from build123d import *
from build123d.topology import SkipClean

# Parameters (mm, degrees)
SKETCH1_R               = 21
BOSS_EXTRUDE1_DEPTH     = 1.5
SKETCH2_R               = 2.65
CUT_EXTRUDE1_DEPTH      = 1.5
SKETCH5_W               = 10
SKETCH5_H               = 30
BOSS_EXTRUDE2_DEPTH     = 1.5
CIRPATTERN1_DEPTH       = 1.5
CUT_EXTRUDE4_REACH      = 38.65
SKETCH4_R               = 1.65
CUT_EXTRUDE5_REACH      = 38.742
SKETCH6_R               = 1.5
CUT_EXTRUDE6_DEPTH      = 37.650375169
CUT_EXTRUDE6_DEPTH_BACK = 37.650375169


# Read off the part's stored shape, not the designer's step: CirPattern1
with BuildPart() as part:
    # Sketch1 → Boss-Extrude1 (new, symmetric)
    with BuildSketch(Plane(origin=(0, 0, 0), x_dir=(1, 0, 0), z_dir=(0, 1, 0))):
        with Locations(Location((0, 0, 0), (0, 0, 270))):
            Circle(SKETCH1_R)
    extrude(amount=BOSS_EXTRUDE1_DEPTH, both=True)

    # Sketch2 → Cut-Extrude1 (cut)
    with BuildSketch(Plane(origin=(0, 1.5, 0), x_dir=(1, 0, 0), z_dir=(0, 1, 0))):
        with Locations((0, -15)):
            Circle(SKETCH2_R)
        with BuildLine():
            ThreePointArc((-2.65, -15), (0, -12.35), (2.65, -15))
            Line((2.65, -15), (4.067821782, -0.821782178))
            ThreePointArc((4.067821782, -0.821782178), (0, -4.15), (-4.067821782, -0.821782178))
            Line((-4.067821782, -0.821782178), (-2.65, -15))
        make_face()
        with BuildLine():
            ThreePointArc((-4.067821782, -0.821782178), (0, -4.15), (4.067821782, -0.821782178))
            Line((4.067821782, -0.821782178), (4.15, 0))
            ThreePointArc((4.15, 0), (0, 4.15), (-4.15, 0))
            Line((-4.15, 0), (-4.067821782, -0.821782178))
        make_face()
    cut_extrude1 = extrude(amount=-CUT_EXTRUDE1_DEPTH, mode=Mode.SUBTRACT)

    # Sketch5 → Boss-Extrude2 (add, symmetric)
    with BuildSketch(Plane(origin=(0, 0, 0), x_dir=(1, 0, 0), z_dir=(0, 1, 0))):
        with Locations((0, -15)):
            Rectangle(SKETCH5_W, SKETCH5_H)
    extrude(amount=BOSS_EXTRUDE2_DEPTH, both=True)

    # Mirror1: Cut-Extrude1 across plane
    with SkipClean():  # the faces are left unmerged after this step: merging them gives an invalid solid
        add(cut_extrude1.mirror(Plane.XY), mode=Mode.SUBTRACT)

    # CirPattern1 outline → CirPattern1 (cut)
    with BuildSketch(Plane(origin=(0, 0, 0), x_dir=(1, 0, 0), z_dir=(0, 1, 0))):
        with BuildLine():
            Line((3.772727273, -3.772727273), (15, -2.65))
            ThreePointArc((15, -2.65), (17.65, 0), (15, 2.65))
            Line((15, 2.65), (3.772727273, 3.772727273))
            Line((3.772727273, 3.772727273), (4.067821782, 0.821782178))
            ThreePointArc((4.067821782, 0.821782178), (0, -4.15), (-4.067821782, 0.821782178))
            Line((-4.067821782, 0.821782178), (-3.772727273, 3.772727273))
            Line((-3.772727273, 3.772727273), (-15, 2.65))
            ThreePointArc((-15, 2.65), (-17.65, 0), (-15, -2.65))
            Line((-15, -2.65), (-3.772727273, -3.772727273))
            Line((-3.772727273, -3.772727273), (-2.65, -15))
            ThreePointArc((-2.65, -15), (0, -17.65), (2.65, -15))
            Line((2.65, -15), (3.772727273, -3.772727273))
        make_face()
    extrude(amount=CIRPATTERN1_DEPTH, mode=Mode.SUBTRACT)

    # Sketch4 → Cut-Extrude4 (cut, up to next)
    with BuildSketch(Plane(origin=(0, 0, 0), x_dir=(1, 0, 0), z_dir=(0, 1, 0)), mode=Mode.PRIVATE) as cut_extrude4_sk1:
        with Locations(Location((0, 0, 0), (0, 0, 270))):
            Circle(SKETCH4_R)
    cut_extrude4_tool1 = extrude(cut_extrude4_sk1.sketch, amount=-CUT_EXTRUDE4_REACH, mode=Mode.PRIVATE) & part.part
    add(cut_extrude4_tool1.solids().sort_by_distance((0, 0, 0))[0], mode=Mode.SUBTRACT)

    # Sketch6 → Cut-Extrude5 (cut, up to next)
    with BuildSketch(Plane(origin=(0, 1.5, 0), x_dir=(1, 0, 0), z_dir=(0, 1, 0)), mode=Mode.PRIVATE) as cut_extrude5_sk1:
        with Locations(Location((2.5, -25.5, 0), (0, 0, 270))):
            Circle(SKETCH6_R)
    cut_extrude5_tool1 = extrude(cut_extrude5_sk1.sketch, amount=-CUT_EXTRUDE5_REACH, mode=Mode.PRIVATE) & part.part
    # Sketch6 → Cut-Extrude5 (cut, up to next)
    with BuildSketch(Plane(origin=(0, 1.5, 0), x_dir=(1, 0, 0), z_dir=(0, 1, 0)), mode=Mode.PRIVATE) as cut_extrude5_sk2:
        with Locations(Location((-2.5, -25.5, 0), (0, 0, 270))):
            Circle(SKETCH6_R)
    cut_extrude5_tool2 = extrude(cut_extrude5_sk2.sketch, amount=-CUT_EXTRUDE5_REACH, mode=Mode.PRIVATE) & part.part
    add(cut_extrude5_tool1.solids().sort_by_distance((2.5, 1.5, 25.5))[0], mode=Mode.SUBTRACT)
    add(cut_extrude5_tool2.solids().sort_by_distance((-2.5, 1.5, 25.5))[0], mode=Mode.SUBTRACT)

    # Sketch7 → Cut-Extrude6 (cut, two sides: drawn at the far end of the back side and taken through both)
    with BuildSketch(Plane(origin=(0, 0, 0), x_dir=(1, 0, 0), z_dir=(0, 1, 0)).offset(-CUT_EXTRUDE6_DEPTH_BACK)):
        with BuildLine():
            ThreePointArc((5, -20.396078054), (0, 21), (-5, -20.396078054))
            Line((-5, -20.396078054), (-5.519486194, -16.207382355))
            ThreePointArc((-5.519486194, -16.207382355), (-5.607043009, -15.695391034), (-5.647210443, -15.177522436))
            Line((-5.647210443, -15.177522436), (-6.513602442, -6.513602442))
            Line((-6.513602442, -6.513602442), (-15.177522436, -5.647210443))
            ThreePointArc((-15.177522436, -5.647210443), (-20.65, 0), (-15.177522436, 5.647210443))
            Line((-15.177522436, 5.647210443), (-6.513602442, 6.513602442))
            Line((-6.513602442, 6.513602442), (-5.647210443, 15.177522436))
            ThreePointArc((-5.647210443, 15.177522436), (0, 20.65), (5.647210443, 15.177522436))
            Line((5.647210443, 15.177522436), (6.513602442, 6.513602442))
            Line((6.513602442, 6.513602442), (15.177522436, 5.647210443))
            ThreePointArc((15.177522436, 5.647210443), (20.65, 0), (15.177522436, -5.647210443))
            Line((15.177522436, -5.647210443), (6.513602442, -6.513602442))
            Line((6.513602442, -6.513602442), (5.647210443, -15.177522436))
            ThreePointArc((5.647210443, -15.177522436), (5.607043009, -15.695391034), (5.519486194, -16.207382355))
            Line((5.519486194, -16.207382355), (5, -20.396078054))
        make_face()
    extrude(amount=CUT_EXTRUDE6_DEPTH + CUT_EXTRUDE6_DEPTH_BACK, mode=Mode.SUBTRACT)


solid = part.part
Can you work these out from the model? Positions are in its coordinate system, mm. A direction names the side the tool comes from. Round coordinates to 2 decimals unless told otherwise and drop trailing zeros. Order: outer loops, then holes, each group sorted by start corner. A loop starts at its lowest first (then second) coordinate and runs counter-clockwise, first axis right, second up. Notation, with made-up numbers: (53, 84.5) -> (103, 84.5) arc R7 ccw to (103, 91.5) -> close; hole circle Ø11 at (15.25, 63.25). An arc over 180 degrees is marked (long way). Write each question's results on one line, items separated by ' | '. Start each with the question number.
Item 1: Thinking about a two-plate mould opening in X: for faces 1 (the flat face through (-10.785, -0.021, 6.086)), 2 (the flat face through (0, 0, 30)), 3 (the flat face through (5.263, -0.021, 18.272)), 4 (the flat face through (-9.31, 0.74, -3.22)), which applies, +X half, -X half, draft (parallel to the pull), parting line (faces both ways), or undercut?
Item 2: Please list where these lines run through material, in increasing order: L1, parallel to X at y = 0.25, z = 25.5; L2, parallel to X at y = 0.85, z = 26; L3, parallel to Z at x = -10, y = 0.75.
Item 3: Which directions (+Z, -Z, +X, -X, +Y, -Y) give clear straight access to the entire face, cutting with the end or side of a thin tool? Please do faces 5 (the flat face through (9.5, 0.7, -3.2)), 6 (the flat face through (5, 0, 25)), 7 (the flat face through (-5, 0, 25)).
Item 4: If we section it at A-A, the plane z = 0: Write out the boundary of the cut face in (x, y), then the cut area to 3 significant figures.
Item 5: If we section it at C-C, the plane x = 0: Write out the boundary of the cut face in (y, z).
Item 6: Will these pins go through, and if not, where does the flat tip stop? pin 1 (1.5 mm diameter, centred on y = -0.5, z = 1, fed in from -X); pin 2 (1.5 mm diameter, centred on y = 0.5, z = 26, fed in from -X).
Item 7: If we section it at B-B, the plane y = 0.6: State how many separate pieces and enclosed holes the cut face has, then the cut area to 3 significant figures.
Item 8: If we section it at D-D, the plane z = 25.5: Write out the boundary of the cut face in (x, y), then the cut area to 3 significant figures.
Results:
1) face 1: -X half | face 2: draft | face 3: +X half | face 4: undercut
2) L1: x = -5 to -4, -1 to 1, 4 to 5 | L2: x = -5 to -3.91, -1.09 to 1.09, 3.91 to 5 | L3: z = -6.16 to -3.15, 3.15 to 6.16
3) face 5: +Y | face 6: +Z, +X, +Y, -Y | face 7: +Z, -X, +Y, -Y
4) outline: (-20.65, -1.5) -> (-1.65, -1.5) -> (-1.65, 0) -> (-17.65, 0) -> (-17.65, 1.5) -> (-20.65, 1.5) -> close; (1.65, -1.5) -> (20.65, -1.5) -> (20.65, 1.5) -> (17.65, 1.5) -> (17.65, 0) -> (1.65, 0) -> close | area: 66.0 mm2
5) outline: (-1.5, -20.65) -> (1.5, -20.65) -> (1.5, -17.65) -> (0, -17.65) -> (0, -1.65) -> (-1.5, -1.65) -> close; (-1.5, 1.65) -> (0, 1.65) -> (0, 17.65) -> (1.5, 17.65) -> (1.5, 30) -> (-1.5, 30) -> close
6) pin 1: stops at x = -20.64 | pin 2: stops at x = -5
7) separate pieces: 1 | enclosed holes: 3 | area: 484 mm2
8) outline: (-5, -1.5) -> (-4, -1.5) -> (-4, 1.5) -> (-5, 1.5) -> close; (-1, -1.5) -> (1, -1.5) -> (1, 1.5) -> (-1, 1.5) -> close; (4, -1.5) -> (5, -1.5) -> (5, 1.5) -> (4, 1.5) -> close | area: 12.0 mm2
